from build123d import *

# Parameters (mm, degrees)
EXTRUDE_1_DEPTH        = 6
SKETCH_2_R             = 1.5
EXTRUDE_2_DEPTH        = 6
HOLE_WIZARD_M3_1_D     = 2.5
HOLE_WIZARD_M3_1_DEPTH = 5
HOLE_WIZARD_M3_1_TIP   = 0.751075774
CHAMFER_1_SIZE         = 0.3


with BuildPart() as part:
    # 草图1 → 凸台-拉伸1 (new body)
    with BuildSketch(Plane.XY):
        Polygon((-1.553072224, 2.69), (-3.106144448, 0), (-1.553072224, -2.69), (1.553072224, -2.69), (3.106144448, 0), (1.553072224, 2.69), align=None)
    extrude(amount=EXTRUDE_1_DEPTH)

    # 草图2 → 凸台-拉伸2 (add)
    with BuildSketch(Plane.XY.offset(6)):
        Circle(SKETCH_2_R)
    extrude(amount=EXTRUDE_2_DEPTH)

    # M3 螺纹孔1
    with Locations(Plane(origin=(0, 0, 0), x_dir=(-1, 0, 0), z_dir=(0, 0, -1))):
        with Locations((0, 0)):
            Hole(HOLE_WIZARD_M3_1_D / 2, depth=HOLE_WIZARD_M3_1_DEPTH)
            with Locations((0, 0, -(HOLE_WIZARD_M3_1_DEPTH + HOLE_WIZARD_M3_1_TIP / 2))):  # 118° drill point
                Cone(0, HOLE_WIZARD_M3_1_D / 2, HOLE_WIZARD_M3_1_TIP, mode=Mode.SUBTRACT)

    # 倒角1
    chamfer_1_edges = [part.edges().sort_by_distance(p)[0] for p in [
        (-1.5, 0, 12),
    ]]
    chamfer(chamfer_1_edges, length=CHAMFER_1_SIZE)


solid = part.part
Verification items for the finished model (mm, model axes). A direction names the side the tool comes from. Give positions to 0.01 mm unless a question says otherwise; leave off trailing zeros. Loops run counter-clockwise (first coordinate to the right, second up) from the corner with the lowest first, then second, coordinate; pieces in that order, holes last. Notation, with made-up numbers: (89, 14.5) - (117, 14.5) arc R17 cw to (117, 28.5) - close; hole circle Ø3 at (89.5, -25.5). An arc over 180 degrees is marked (long way). Write each question's results on one line, items separated by ' | '.
1) Sectioned sample at A-A on z = 4.75. Record the boundary of the cut face in (x, y).
Solution:
outline: (-3.11, 0) - (-1.55, -2.69) - (1.55, -2.69) - (3.11, 0) - (1.55, 2.69) - (-1.55, 2.69) - close; hole circle Ø2.5 at (0, 0)
2) Material ranges on L1, parallel to Y at x = 0, z = 4; L2, parallel to Z at x = 1, y = -2.2; L3, parallel to X at y = 0.9, z = 2.25, recorded low to high. Write a range as from..to.
Solution:
L1: -2.69..-1.25, 1.25..2.69 | L2: 0..6 | L3: -2.59..-0.87, 0.87..2.59
3) Tool access check on faces 4 (the flat face through (2.3, -1.4, 3)), 5 (the flat face through (1.3, 1.2, 6)). Record the directions out of +Z, -Z, +X, -X, +Y, -Y that give a thin tool (end or side, any length) a straight path to the whole face; none if there is none.
Solution:
face 4: +Z, -Z, +X, -Y | face 5: +Z
4) Sectioned sample at B-B on z = 11.25. Record the boundary of the cut face in (x, y), plus the area to 3 significant figures.
Solution:
outline: circle Ø3 at (0, 0) | area: 7.07 mm2
5) Sectioned sample at C-C on y = 1.85. Record the boundary of the cut face in (x, z), plus the area to 3 significant figures.
Solution:
outline: (-2.04, 0) - (2.04, 0) - (2.04, 6) - (-2.04, 6) - close | area: 24.5 mm2
6) Sectioned sample at D-D on x = 2. Record the boundary of the cut face in (y, z), plus the area to 3 significant figures.
Solution:
outline: (-1.92, 0) - (1.92, 0) - (1.92, 6) - (-1.92, 6) - close | area: 23.0 mm2
7) Mould release check, pull along X, two halves, no side actions. Record for faces 1 (the cylindrical face through (-0.27, -1.22, 2.54)), 2 (the cylindrical face through (-1.5, 0.07, 8.81)), 3 (the flat face through (1, -1, 0)): pulls with the +X half, pulls with the -X half, needs draft (parallel to the pull), parting line crosses it, or undercut.
Solution:
face 1: undercut | face 2: parting line crosses it | face 3: needs draft
